For this review, take the finished solid that the model builds, in its own axes (mm). Give positions to 0.01 mm unless a question says otherwise; leave off trailing zeros. Write each loop counter-clockwise with the first axis right and the second up, starting at its lowest first coordinate (ties: lowest second). Pieces come first, ordered by that corner, then holes.
Q1. We need section C-C (z = 37.5). Write out the cut boundary in (x, y), then the cut area to 3 significant figures.
Q2. For line 1 (Y direction, x = -349, z = -39); line 2 (Y direction, x = 257, z = -20.5); line 3 (Y direction, x = 204.5, z = -36), list the stretches that pass through material, from the lowest coordinate up.
Q3. Mouldability with a two-part tool opening along Y and no side actions: class faces 1 (the flat face through (-318, -12.7, -51)), 2 (the flat face through (-372, -63.5, -51)), 3 (the flat face through (-318, -38.1, -51)) as released by +Y, released by -Y, zero draft, split by the parting line, or undercut.
Q4. Insertion check: P1, Ø8, axis at x = 229, y = -31, coming from the +Z side; P2, Ø6.5, axis at x = -370, y = -30.5, coming from the +Z side; P3, Ø4, axis at y = -9, z = 0, coming from the +X side. Each pin has a flat end and moves straight along its axis. Give the tip position at first contact, or say it passes through.
Q5. We need section A-A (x = 204). Write out the cut boundary in (y, z), then the cut area to 3 significant figures.
Q6. We need section B-B (x = 349). Write out the cut boundary in (y, z), then the cut area to 3 significant figures.
```python
from build123d import *

# Parameters (mm, degrees)
F0_W      = 914.4
F0_H      = 152.4
F1_DEPTH  = 63.5
F2_R      = 6.35
F2_W      = 25.4
F2_H      = 19.05
F2_W_2    = 154.94
F2_H_2    = 25.4
F2_W_3    = 101.6
F2_H_3    = 12.7
F2_W_4    = 63.5
F2_W_5    = 203.2
F2_H_4    = 44.45
F2_H_5    = 21.59
F3_DEPTH  = 139.7
F4_W      = 120.65
F4_H      = 63.5
F5_DEPTH  = 88.9
F6_W      = 101.6
F6_H      = 63.5
F7_DEPTH  = 114.3
F8_W      = 247.65
F8_H      = 63.5
F9_DEPTH  = 107.95
F10_W     = 227.33
F10_H     = 63.5
F11_DEPTH = 88.9
F12_W     = 217.17
F12_H     = 50.8
F13_DEPTH = 152.4


with BuildPart() as f1:
    # F0 (on Front) → F1 (new body)
    with BuildSketch(Plane.XZ):
        Rectangle(F0_W, F0_H)
    extrude(amount=F1_DEPTH)

    # F2 (on face) → F3 (cut)
    with BuildSketch(Plane.XY.offset(76.2)):
        with Locations((-444.5, -12.7)):
            Circle(F2_R)
        with Locations((-425.45, -12.7)):
            Circle(F2_R)
        with Locations((-406.4, -12.7)):
            Circle(F2_R)
        with Locations((-387.35, -12.7)):
            Circle(F2_R)
        with Locations((-368.3, -12.7)):
            Circle(F2_R)
        with Locations((-349.25, -12.7)):
            Circle(F2_R)
        with Locations((-444.5, -31.75)):
            Circle(F2_R)
        with Locations((-425.45, -31.75)):
            Circle(F2_R)
        with Locations((-406.4, -31.75)):
            Circle(F2_R)
        with Locations((-387.35, -31.75)):
            Circle(F2_R)
        with Locations((-368.3, -31.75)):
            Circle(F2_R)
        with Locations((-349.25, -31.75)):
            Circle(F2_R)
        with Locations((-444.5, -50.8)):
            Circle(F2_R)
        with Locations((-425.45, -50.8)):
            Circle(F2_R)
        with Locations((-406.4, -50.8)):
            Circle(F2_R)
        with Locations((-387.35, -50.8)):
            Circle(F2_R)
        with Locations((-368.3, -50.8)):
            Circle(F2_R)
        with Locations((-349.25, -50.8)):
            Circle(F2_R)
        with Locations((-317.5, -47.625)):
            Rectangle(F2_W, F2_H)
        with Locations((-317.5, -22.225)):
            Rectangle(F2_W, F2_H)
        with Locations((-285.75, -22.225)):
            Rectangle(F2_W, F2_H)
        with Locations((-285.75, -47.625)):
            Rectangle(F2_W, F2_H)
        with Locations((-254, -22.225)):
            Rectangle(F2_W, F2_H)
        with Locations((-254, -47.625)):
            Rectangle(F2_W, F2_H)
        with Locations((64.77, -25.4)):
            Rectangle(F2_W_2, F2_H_2)
        with Locations((64.77, -50.8)):
            Rectangle(F2_W_3, F2_H_3)
        with Locations((186.69, -19.05)):
            Rectangle(F2_W_4, F2_H_2)
        with Locations((345.44, -28.575)):
            Rectangle(F2_W_5, F2_H_4)
        with Locations((186.69, -46.355)):
            Rectangle(F2_W_4, F2_H_5)
    extrude(amount=-F3_DEPTH, mode=Mode.SUBTRACT)

    # F4 (on face) → F5 (cut)
    with BuildSketch(Plane.XY.offset(76.2)):
        with Locations((-396.875, -31.75)):
            Rectangle(F4_W, F4_H)
    extrude(amount=-F5_DEPTH, mode=Mode.SUBTRACT)

    # F6 (on face) → F7 (cut)
    with BuildSketch(Plane.XY.offset(76.2)):
        with Locations((-285.75, -31.75)):
            Rectangle(F6_W, F6_H)
    extrude(amount=-F7_DEPTH, mode=Mode.SUBTRACT)

    # F8 (on face) → F9 (cut)
    with BuildSketch(Plane.XY.offset(76.2)):
        with Locations((106.045, -31.75)):
            Rectangle(F8_W, F8_H)
    extrude(amount=-F9_DEPTH, mode=Mode.SUBTRACT)

    # F10 (on face) → F11 (cut)
    with BuildSketch(Plane.XY.offset(76.2)):
        with Locations((343.535, -31.75)):
            Rectangle(F10_W, F10_H)
    extrude(amount=-F11_DEPTH, mode=Mode.SUBTRACT)

    # F12 (on face) → F13 (cut)
    with BuildSketch(Plane.XY.offset(76.2)):
        with Locations((-126.365, -38.1)):
            Rectangle(F12_W, F12_H)
    extrude(amount=-F13_DEPTH, mode=Mode.SUBTRACT)


solid = f1.part
```
Computed:
1. outline: (-234.95, -12.7) - (-17.78, -12.7) - (-17.78, 0) - (-234.95, 0) - close
1. area: 2,760 mm2
2. line 1: y = -63.5 to -57.15, -44.45 to -38.1, -25.4 to -19.05, -6.35 to 0
2. line 2: y = -63.5 to -50.8, -6.35 to 0
2. line 3: y = -63.5 to -57.15, -35.56 to -31.75, -6.35 to 0
3. face 1: undercut
3. face 2: released by -Y
3. face 3: undercut
4. P1: stops at z = -12.7
4. P2: stops at z = -63.5
4. P3: stops at x = -17.78
5. outline: (-63.5, -76.2) - (0, -76.2) - (0, -31.75) - (-6.35, -31.75) - (-6.35, -63.5) - (-31.75, -63.5) - (-31.75, -31.75) - (-35.56, -31.75) - (-35.56, -63.5) - (-57.15, -63.5) - (-57.15, -31.75) - (-63.5, -31.75) - close
5. area: 1,330 mm2
6. outline: (-63.5, -76.2) - (0, -76.2) - (0, -12.7) - (-6.35, -12.7) - (-6.35, -63.5) - (-50.8, -63.5) - (-50.8, -12.7) - (-63.5, -12.7) - close
6. area: 1,770 mm2
